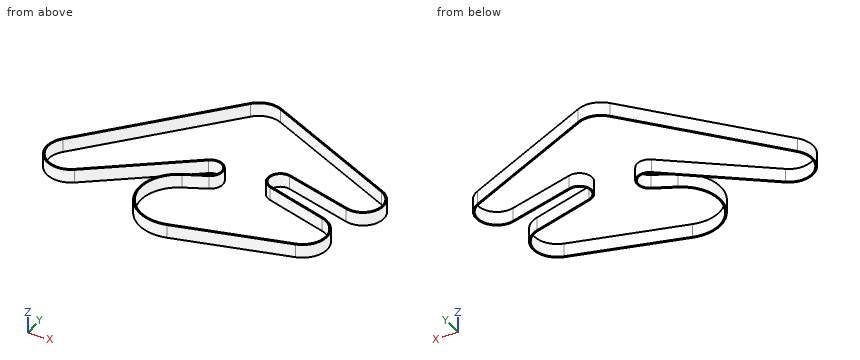
from build123d import *

# Parameters (mm, degrees)
EXTRUDE_THIN1_DEPTH = 18


with BuildPart() as part:
    # Sketch1 → Extrude-Thin1 (new body)
    with BuildSketch(Plane.XY):
        with BuildLine():
            Line((6.327716808, 61.4), (-22.357932721, 48.053333333))
            ThreePointArc((-22.357932721, 48.053333333), (-49.857891872, -17.97750311), (13.453428864, -51.264073695))
            Line((13.453428864, -51.264073695), (163.376663255, -11.919140225))
            ThreePointArc((163.376663255, -11.919140225), (187.995352271, 19.446169247), (164.443175515, 51.620032198))
            Line((164.443175515, 51.620032198), (80.707647493, 76.627258092))
            ThreePointArc((80.707647493, 76.627258092), (70.593974061, 95.179284225), (89.0659579, 105.438420494))
            Line((89.0659579, 105.438420494), (178.940955528, 80.129006849))
            ThreePointArc((178.940955528, 80.129006849), (212.749176963, 97.252513036), (198.527826902, 132.380329695))
            Line((198.527826902, 132.380329695), (14.139419596, 219.817391125))
            ThreePointArc((14.139419596, 219.817391125), (-6.373631689, 222.37864758), (-24.385542849, 212.233877304))
            Line((-24.385542849, 212.233877304), (-179.385542849, 42.233877304))
            ThreePointArc((-179.385542849, 42.233877304), (-179.495266598, -2.112935452), (-135.368386906, -6.525455083))
            Line((-135.368386906, -6.525455083), (-8.923460497, 87.057025038))
            ThreePointArc((-8.923460497, 87.057025038), (12.893998789, 82.664515329), (6.327716808, 61.4))
        make_face()
        with BuildLine():
            Line((7.171412382, 59.586666667), (-21.514237147, 46.24))
            ThreePointArc((-21.514237147, 46.24), (-47.97646199, -17.299106766), (12.945752303, -49.329580348))
            Line((12.945752303, -49.329580348), (162.868986694, -9.984646878))
            ThreePointArc((162.868986694, -9.984646878), (185.995633952, 19.479734747), (163.870861847, 49.70366661))
            Line((163.870861847, 49.70366661), (80.135333826, 74.710892504))
            ThreePointArc((80.135333826, 74.710892504), (68.673170602, 95.736522122), (89.60808562, 107.363543226))
            Line((89.60808562, 107.363543226), (179.483083248, 82.054129582))
            ThreePointArc((179.483083248, 82.054129582), (210.876431723, 97.954528184), (197.670892381, 130.573215081))
            Line((197.670892381, 130.573215081), (13.282485075, 218.010276511))
            ThreePointArc((13.282485075, 218.010276511), (-5.98735098, 220.416305302), (-22.907631161, 210.886369588))
            Line((-22.907631161, 210.886369588), (-177.907631161, 40.886369588))
            ThreePointArc((-177.907631161, 40.886369588), (-178.010704986, -0.772757545), (-136.558181639, -4.917851744))
            Line((-136.558181639, -4.917851744), (-10.11325523, 88.664628376))
            ThreePointArc((-10.11325523, 88.664628376), (14.613198627, 83.686450706), (7.171412382, 59.586666667))
        make_face(mode=Mode.SUBTRACT)
    extrude(amount=EXTRUDE_THIN1_DEPTH)


solid = part.part
Could you check a few things on this model? Use its own coordinates, in mm. Give positions to 0.01 mm unless a question says otherwise; leave off trailing zeros. Order: outer loops, then holes, each group sorted by start corner. A loop starts at its lowest first (then second) coordinate and runs counter-clockwise, first axis right, second up. Notation, with made-up numbers: (71.5, 76) - (79.5, 76) arc R17 ccw to (79.5, 97) - close; hole circle Ø9 at (76.5, 67). An arc over 180 degrees is marked (long way). Return JSON: item names as keys, results as strings. Group by question number.
Q1. Suppose I cut it at C-C, the plane y = -23.5. Please give me the cut outline in (x, z), and give its area (3 significant figures).
Q2. Suppose I cut it at A-A, the plane z = 6. Please give me the cut outline in (x, y), and give its area (3 significant figures).
Q3. Suppose I cut it at B-B, the plane x = -114.5. Please give me the cut outline in (y, z).
Q4. Suppose I cut it at D-D, the plane x = 0. Please give me the cut outline in (y, z).
Q5. Please list where these lines run through material, in increasing order: line 1 along Y through (x, z) = (0, 4); line 2 along Y through (x, z) = (118.5, 3.75); line 3 along X through (y, z) = (3.5, 11). Write a range as [from, to].
Q6. Will these pins go through, and if not, where does the flat tip stop? pin 1 Ø8 at (y, z) = (117, 14.5) entering from +X; pin 2 Ø3 at (x, z) = (49.5, 2.5) entering from +Y; pin 3 Ø8 at (y, z) = (8, 8) entering from -X.
Resolved:
{
 "1": {"outline": "(-47.51, 0) - (-45.26, 0) - (-45.26, 18) - (-47.51, 18) - close; (111.37, 0) - (119.25, 0) - (119.25, 18) - (111.37, 18) - close", "area": "182 mm2"},
 "2": {"outline": "(-179.39, 42.23) arc R33 ccw to (-135.37, -6.53) - (-8.92, 87.06) arc R15 cw (long way) to (6.33, 61.4) - (-22.36, 48.05) arc R53 ccw to (13.45, -51.26) - (163.38, -11.92) arc R33 ccw to (164.44, 51.62) - (80.71, 76.63) arc R15 cw to (89.07, 105.44) - (178.94, 80.13) arc R28 ccw to (198.53, 132.38) - (14.14, 219.82) arc R33 ccw to (-24.39, 212.23) - close; hole (-177.91, 40.89) arc R31 ccw to (-136.56, -4.92) - (-10.11, 88.66) arc R17 cw (long way) to (7.17, 59.59) - (-21.51, 46.24) arc R51 ccw to (12.95, -49.33) - (162.87, -9.98) arc R31 ccw to (163.87, 49.7) - (80.14, 74.71) arc R17 cw to (89.61, 107.36) - (179.48, 82.05) arc R26 ccw to (197.67, 130.57) - (13.28, 218.01) arc R31 ccw to (-22.91, 210.89) - close", "area": "3,030 mm2"},
 "3": {"outline": "(8.92, 0) - (11.41, 0) - (11.41, 18) - (8.92, 18) - close; (110.43, 0) - (113.4, 0) - (113.4, 18) - (110.43, 18) - close"},
 "4": {"outline": "(-53, 0) - (-51, 0) - (-51, 18) - (-53, 18) - close; (56.25, 0) - (58.46, 0) - (58.46, 18) - (56.25, 18) - close; (90, 0) - (92, 0) - (92, 18) - (90, 18) - close; (221, 0) - (223, 0) - (223, 18) - (221, 18) - close"},
 "5": {"line 1": "y = [-53, -51], [56.25, 58.46], [90, 92], [221, 223]", "line 2": "y = [-23.7, -21.63], [63.25, 65.34], [97.15, 99.23], [168.12, 170.33]", "line 3": "x = [-183.58, -181.24], [-125.18, -121.82], [-52.88, -50.88], [181.24, 183.58]"},
 "6": {"pin 1": "stops at x = 213.9", "pin 2": "stops at y = 203.76", "pin 3": "stops at x = -187.02"}
}
